Geometry: see drawing. Coordinates: mm, zero at the bounding-box minimum. A direction names the side the tool comes from. Round coordinates to 2 decimals unless told otherwise and drop trailing zeros. Loops run counter-clockwise (first coordinate to the right, second up) from the corner with the lowest first, then second, coordinate; pieces in that order, holes last. Notation, with made-up numbers: M 23.25,7.5 L 42.25,7.5 A10 cw 42.25,19.5 Z; hole C 55,-1 d10. An arc over 180 degrees is marked long. Answer as a JSON object with one key per item and string values.
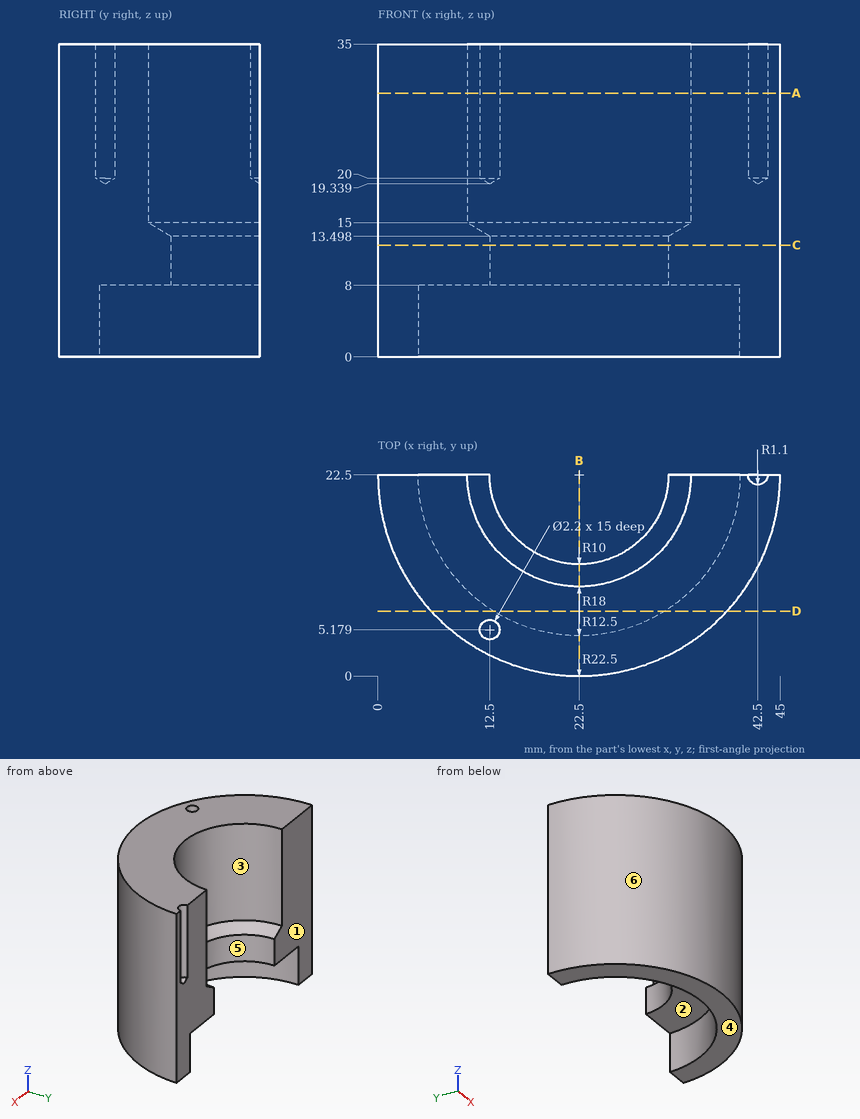
1) Pull-direction query (X, two-part tool) for the marked faces 4, 5 and 6; classes: +X half, -X half, draft (parallel to the pull), parting line (faces both ways), or undercut.
Results:
{"face 4": "draft", "face 5": "undercut", "face 6": "parting line"}
2) Section query D-D (y = 7.25). Return the cut outline in (x, z), and give its area (4 significant figures).
Results:
{"outline": "M 5.96,0 L 12.94,0 L 12.94,8 L 32.06,8 L 32.06,0 L 39.04,0 L 39.04,35 L 5.96,35 Z", "area": "1,005 mm2"}
3) Section query C-C (z = 12.5). Return the cut outline in (x, y).
Results:
{"outline": "M 0,22.5 A22.5 ccw 45,22.5 L 32.5,22.5 A10 cw 12.5,22.5 Z"}
4) Section query B-B (x = 22.5). Return the cut outline in (y, z).
Results:
{"outline": "M 0,0 L 4.5,0 L 4.5,8 L 12.5,8 L 12.5,13.5 L 10,15 L 10,35 L 0,35 Z"}
5) Pin query (flat end, axial travel): P1, Ø6, axis at x = 32.5, z = 5, coming from the -Y side; P2, Ø12, axis at x = 28, y = 19, coming from the -Z side; P3, Ø2, axis at x = 12.5, y = 5.18, coming from the -Z side; P4, Ø6, axis at x = 21.5, z = 5, coming from the -Y side. Return the tip coordinate at first contact, or that it passes through.
Results:
{"P1": "y = 1.12", "P2": "z = 8", "P3": "z = 0", "P4": "y = 0"}
6) Ray query, line 1 (X direction, y = 21.5, z = 24) (1 decimal); line 2 (Z direction, x = 19.5, y = 7.25); line 3 (X direction, y = 16.25, z = 27) (1 decimal). Return the intervals inside material, ascending.
Results:
{"line 1": "0 to 10, 35 to 42, 43 to 45", "line 2": "8 to 35", "line 3": "0.9 to 11.7, 33.3 to 44.1"}
7) Section query A-A (z = 29.5). Return the cut outline in (x, y), and give its area (3 significant figures).
Results:
{"outline": "M 0,22.5 A22.5 ccw 45,22.5 L 43.6,22.5 A1.1 cw 41.4,22.5 L 35,22.5 A12.5 cw 10,22.5 Z; hole C 12.5,5.18 d2.2", "area": "544 mm2"}
8) Reachability of the marked faces 1, 2 and 3 from +Z, -Z, +X, -X, +Y, -Y: full face, straight path, thin tool, end or side. Return the list, or none.
Results:
{"face 1": "+Z, -Z, +X, -X, +Y", "face 2": "-Z, +Y", "face 3": "+Z, +Y"}
